Geometry check sheet. Reference: the model listing, model coordinates, mm. Give positions to 0.01 mm unless a question says otherwise; leave off trailing zeros. Loops run counter-clockwise (first coordinate to the right, second up) from the corner with the lowest first, then second, coordinate; pieces in that order, holes last. Notation, with made-up numbers: (77.25, 82) -> (86.25, 82) arc R22 cw to (86.25, 99) -> close; hole circle Ø6 at (43.25, 30.25). An arc over 180 degrees is marked (long way). Write each question's results on one line, items separated by ' | '. Start each with the question number.
1) Scan lines: line 1 (Z direction, x = 6.75, y = -1.5); line 2 (Z direction, x = -6.5, y = 3.5); line 3 (X direction, y = -3.25, z = 0.05). Record each from-to range of solid material in increasing order. Write a range as from..to.
2) Sectioned sample at C-C on z = 0.3. Record the cut outline in (x, y), then the cut area to 3 significant figures.
3) Depth check by flat-ended pin: pin 1 (1.4 mm diameter, centred on x = -1, y = -3.5, fed in from -Z). Enter the tip coordinate at first touch or a pass-through.
```python
from build123d import *

# Parameters (mm, degrees)
SKETCH1_W           = 24
SKETCH1_H           = 8.2
BOSS_EXTRUDE1_DEPTH = 1.5
SKETCH2_W           = 24
SKETCH2_H           = 2.4
BOSS_EXTRUDE2_DEPTH = 1.4
BOSS_EXTRUDE2_DRAFT = -10
FILLET1_R           = 1.5


with BuildPart() as part:
    # Sketch1 → Boss-Extrude1 (new body)
    with BuildSketch(Plane.XY):
        Rectangle(SKETCH1_W, SKETCH1_H)
    extrude(amount=BOSS_EXTRUDE1_DEPTH)


with BuildPart() as boss_extrude2_tool:
    # Sketch2 → Boss-Extrude2 (with draft: the straight prism first)
    with BuildSketch(Plane(origin=(0, 0, 0), x_dir=(-1, 0, 0), z_dir=(0, 0, -1))):
        Rectangle(SKETCH2_W, SKETCH2_H)
    extrude(amount=BOSS_EXTRUDE2_DEPTH)
    # Boss-Extrude2: the draft: its side faces are tilted about the plane it starts from
    boss_extrude2_sides = [boss_extrude2_tool.faces().sort_by_distance(p)[0] for p in [
        (12, 0, -0.7),
        (0, -1.2, -0.7),
        (-12, 0, -0.7),
        (0, 1.2, -0.7),
    ]]
    draft(boss_extrude2_sides, Plane(origin=(0, 0, 0), x_dir=(-1, 0, 0), z_dir=(0, 0, -1)), BOSS_EXTRUDE2_DRAFT)


with BuildPart() as part_1:
    add(part.part)

    # Boss-Extrude2: add boss_extrude2_tool
    add(boss_extrude2_tool.part)

    # Fillet1
    fillet1_edges = [part_1.edges().sort_by_distance(p)[0] for p in [
        (0, -4.1, 1.5),
        (-12, 0, 1.5),
        (0, 4.1, 1.5),
        (12, 0, 1.5),
    ]]
    fillet(fillet1_edges, radius=FILLET1_R - 0.0001)  # a hair under: the kernel refuses the full size


solid = part_1.part
```
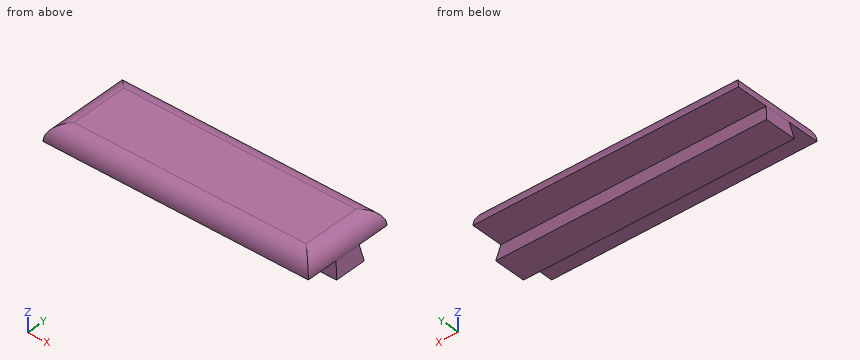
Result:
1) line 1: 0..1.5 | line 2: 0..1.2 | line 3: -12..12
2) outline: (-11.97, -4.07) -> (11.97, -4.07) -> (11.97, 4.07) -> (-11.97, 4.07) -> close | area: 195 mm^2
3) pin 1: z = 0
